from build123d import *

# Parameters (mm, degrees)
SKETCH1_W           = 50
SKETCH1_H           = 35.56
SKETCH1_R           = 11
BOSS_EXTRUDE1_DEPTH = 49
SKETCH2_W           = 31.5
SKETCH2_H           = 32.56
BOSS_EXTRUDE2_DEPTH = 2
SKETCH3_W           = 0.8
SKETCH3_H           = 6
BOSS_EXTRUDE3_DEPTH = 15
CHAMFER1_SIZE       = 1


with BuildPart() as part:
    # Sketch1 → Boss-Extrude1 (new body)
    with BuildSketch(Plane.XY):
        Rectangle(SKETCH1_W, SKETCH1_H)
        with Locations((-3, 0)):
            Circle(SKETCH1_R, mode=Mode.SUBTRACT)
    extrude(amount=BOSS_EXTRUDE1_DEPTH)

    # Sketch2 → Boss-Extrude2 (add)
    with BuildSketch(Plane(origin=(25, 0, 0), x_dir=(0, 0, -1), z_dir=(1, 0, 0))):
        with Locations((-17.25, 0)):
            Rectangle(SKETCH2_W, SKETCH2_H)
    extrude(amount=BOSS_EXTRUDE2_DEPTH)

    # Sketch3 → Boss-Extrude3 (add)
    with BuildSketch(Plane(origin=(27, 0, 0), x_dir=(0, 0, -1), z_dir=(1, 0, 0))):
        Polygon((-16.5, 5), (-16.5, 8), (-12.5, 8), (-12.5, 5), (-11.5, 5), (-11.5, 9), (-17.5, 9), (-17.5, 5), align=None)
        with Locations((-6.9, 0)):
            Rectangle(SKETCH3_W, SKETCH3_H)
        Polygon((-12.5, -5), (-11.5, -5), (-11.5, -9), (-17.5, -9), (-17.5, -5), (-16.5, -5), (-16.5, -8), (-12.5, -8), align=None)
    extrude(amount=BOSS_EXTRUDE3_DEPTH)

    # Chamfer1
    chamfer1_edges = [part.edges().sort_by_distance(p)[0] for p in [
        (0, 17.78, 49),
        (-25, 0, 49),
        (0, 17.78, 0),
        (0, -17.78, 0),
        (-25, 0, 0),
        (0, -17.78, 49),
    ]]
    chamfer(chamfer1_edges, length=CHAMFER1_SIZE)


solid = part.part
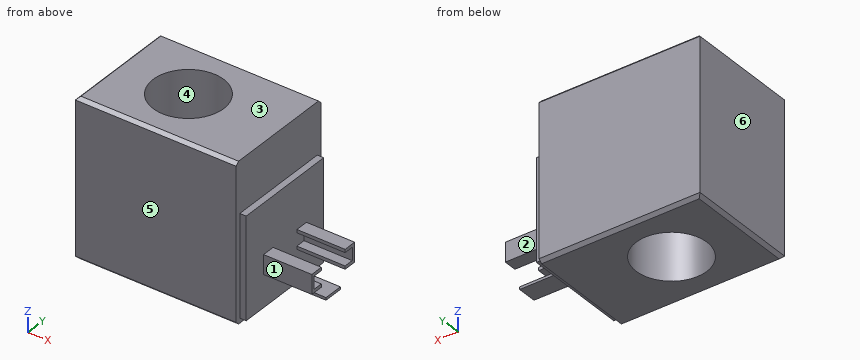
For this review, take the finished solid that the model builds, in its own axes (mm). Face numbers are marked on the shaded views. A direction names the side the tool comes from. Round coordinates to 2 decimals unless told otherwise and drop trailing zeros. Write each loop counter-clockwise with the first axis right and the second up, starting at its lowest first coordinate (ties: lowest second). Pieces come first, ordered by that corner, then holes. Notation, with made-up numbers: M 85.25,65.25 L 109.25,65.25 A11 cw 109.25,81.25 Z; hole C -29,7.25 d3. An arc over 180 degrees is marked long. Write item = value, one per line. Start each with the question number.
(1) The part is to be moulded in two halves that separate along X. For the marked faces 4, 5 and 6, say which applies: +X half, -X half, draft (parallel to the pull), parting line (faces both ways), or undercut.
(2) We need section B-B (x = -3). Give the boundary of the cut face in (y, z).
(3) We need section C-C (z = 27.5). Give the boundary of the cut face in (x, y), then the cut area to 3 significant figures.
(4) For line 1 along Y through (x, z) = (-3, 38.5); line 2 along X through (y, z) = (-1, 21.5); line 3 along X through (y, z) = (-5.5, 36.5), list the stretches that pass through material, from the lowest coordinate up.
(5) For the marked faces 1, 2 and 3, list the 3-axis set-ups (+Z, -Z, +X, -X, +Y, -Y) from which the entire face can be reached by the end or side of a thin tool; tool diameter is ignored.
(6) We need section A-A (y = 0). Give the boundary of the cut face in (x, z), then the cut area to 3 significant figures.
(7) Clearance check with flat-ended pins moving along their axes: pin 1 Ø1.6 at (x, y) = (26, -2) entering from -Z; pin 2 Ø4 at (y, z) = (-6, 36) entering from +X; pin 3 Ø0.8 at (x, z) = (35, 12) entering from +Y. State where each tip first meets the part, or that it passes through.
(8) We need section D-D (y = 15). Give the boundary of the cut face in (x, z).
Results found:
q1.face_4 = undercut
q1.face_5 = draft
q1.face_6 = -X half
q2.outline = M -17.78,1 L -16.78,0 L -11,0 L -11,49 L -16.78,49 L -17.78,48 Z; M 11,0 L 16.78,0 L 17.78,1 L 17.78,48 L 16.78,49 L 11,49 Z
q3.outline = M -25,-17.78 L 25,-17.78 L 25,-16.28 L 27,-16.28 L 27,16.28 L 25,16.28 L 25,17.78 L -25,17.78 Z; hole C -3,0 d22
q3.area = 1,460 mm²
q4.line_1 = -17.78 to -11, 11 to 17.78
q4.line_2 = -25 to -13.95, 7.95 to 27
q4.line_3 = -25 to -12.53, 6.53 to 25
q5.face_1 = +Z, -Z, +X, -Y
q5.face_2 = +Z, -Z, +X, +Y
q5.face_3 = +Z, +X, -X, +Y, -Y
q6.outline = M -25,1 L -24,0 L -14,0 L -14,49 L -24,49 L -25,48 Z; M 8,0 L 25,0 L 25,1.5 L 27,1.5 L 27,6.5 L 42,6.5 L 42,7.3 L 27,7.3 L 27,33 L 25,33 L 25,49 L 8,49 Z
q6.area = 1,450 mm²
q7.pin_1 = 1.5
q7.pin_2 = 25
q7.pin_3 = 9
q8.outline = M -25,1 L -24,0 L 25,0 L 25,1.5 L 27,1.5 L 27,33 L 25,33 L 25,49 L -24,49 L -25,48 Z
